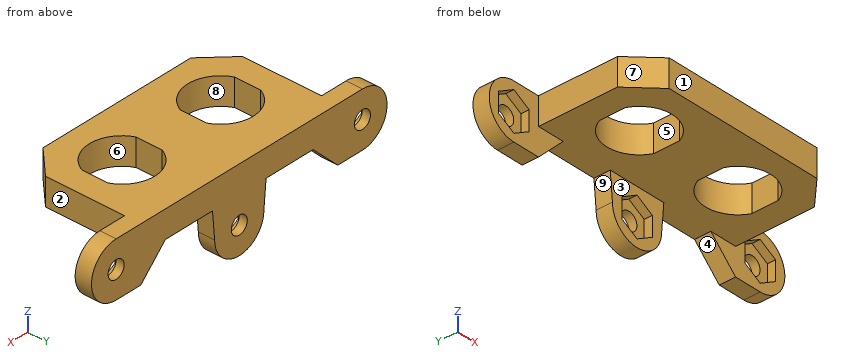
from build123d import *
from OCP.BRepFilletAPI import BRepFilletAPI_MakeChamfer

# Parameters (mm, degrees)
SKETCH1_R           = 1.625
BOSS_EXTRUDE1_DEPTH = 22.5
SKETCH5_W           = 15
SKETCH5_H           = 5
CUT_EXTRUDE1_DEPTH  = 41.388736054
CUT_EXTRUDE2_DEPTH  = 19.5
CUT_EXTRUDE3_DEPTH  = 39.810436741
CHAMFER1_SIZE       = 5
CHAMFER2_SIZE       = 0.437443318
CHAMFER2_SIZE_2     = 5
CHAMFER3_SIZE       = 5
CUT_EXTRUDE4_DEPTH  = 1.5


with BuildPart() as part:
    # Sketch1 → Boss-Extrude1 (new body)
    with BuildSketch(Plane(origin=(0, 0, 0), x_dir=(1, 0, 0), z_dir=(0, 1, 0))):
        with BuildLine():
            Line((-25, 10), (-5, 10))
            ThreePointArc((-5, 10), (0, 15), (5, 10))
            Line((5, 10), (25, 10))
            ThreePointArc((25, 10), (30, 5), (25, 0))
            Line((25, 0), (-25, 0))
            ThreePointArc((-25, 0), (-30, 5), (-25, 10))
        make_face()
        with Locations(Location((-25, 5, 0), (0, 0, 90))):
            Circle(SKETCH1_R, mode=Mode.SUBTRACT)
        with Locations(Location((25, 5, 0), (0, 0, 90))):
            Circle(SKETCH1_R, mode=Mode.SUBTRACT)
        with Locations(Location((0, 10, 0), (0, 0, 90))):
            Circle(SKETCH1_R, mode=Mode.SUBTRACT)
    extrude(amount=BOSS_EXTRUDE1_DEPTH)

    # Sketch5 → Cut-Extrude1 (cut, through all)
    with BuildSketch(Plane(origin=(0, 0, 0), x_dir=(1, 0, 0), z_dir=(0, 1, 0))):
        with Locations((-12.5, 7.5)):
            Rectangle(SKETCH5_W, SKETCH5_H)
        with Locations((12.5, 7.5)):
            Rectangle(SKETCH5_W, SKETCH5_H)
    extrude(amount=CUT_EXTRUDE1_DEPTH, mode=Mode.SUBTRACT)

    # Sketch6 → Cut-Extrude2 (cut)
    with BuildSketch(Plane.XZ):
        with BuildLine():
            Line((-25, 0), (-20, 0))
            Line((-20, 0), (-20, -10))
            Line((-20, -10), (-25, -10))
            ThreePointArc((-25, -10), (-30, -5), (-25, 0))
        make_face()
        with BuildLine():
            Line((20, 0), (20, -10))
            Line((20, -10), (25, -10))
            ThreePointArc((25, -10), (30, -5), (25, 0))
            Line((25, 0), (20, 0))
        make_face()
        with BuildLine():
            Line((-5, -5), (5, -5))
            Line((5, -5), (5, -10))
            ThreePointArc((5, -10), (0, -15), (-5, -10))
            Line((-5, -10), (-5, -5))
        make_face()
    extrude(amount=-CUT_EXTRUDE2_DEPTH, mode=Mode.SUBTRACT)

    # Sketch7 → Cut-Extrude3 (cut, through all)
    with BuildSketch(Plane(origin=(0, 0, -5), x_dir=(-1, 0, 0), z_dir=(0, 0, -1))):
        with BuildLine():
            Line((4.5, 12.397915762), (4.5, 7.602084238))
            ThreePointArc((4.5, 7.602084238), (10, 4), (15.5, 7.602084238))
            Line((15.5, 7.602084238), (15.5, 12.397915762))
            ThreePointArc((15.5, 12.397915762), (10, 16), (4.5, 12.397915762))
        make_face()
        with BuildLine():
            Line((-15.5, 12.397915762), (-15.5, 7.602084238))
            ThreePointArc((-15.5, 7.602084238), (-10, 4), (-4.5, 7.602084238))
            Line((-4.5, 7.602084238), (-4.5, 12.397915762))
            ThreePointArc((-4.5, 12.397915762), (-10, 16), (-15.5, 12.397915762))
        make_face()
    extrude(amount=-CUT_EXTRUDE3_DEPTH, mode=Mode.SUBTRACT)

    # Chamfer1
    chamfer1_edges = [part.edges().sort_by_distance(p)[0] for p in [
        (-20, 21, -5),
        (20, 21, -5),
    ]]
    chamfer(chamfer1_edges, length=CHAMFER1_SIZE - 0.0001)  # a hair under: the kernel refuses the full size

    # Chamfer2
    chamfer2_edges_1 = [part.edges().sort_by_distance(p)[0] for p in [
        (-5, 21, -5),
    ]]
    chamfer2_side_1 = [part.faces().sort_by_distance(p)[0] for p in [
        (-5.008748866, 21, -5),
    ]]
    chamfer2_edges_2 = [part.edges().sort_by_distance(p)[0] for p in [
        (5, 21, -5),
    ]]
    chamfer2_side_2 = [part.faces().sort_by_distance(p)[0] for p in [
        (5.008748866, 21, -5),
    ]]
    chamfer2 = BRepFilletAPI_MakeChamfer(part.part.solid().wrapped)
    for e in chamfer2_edges_1:
        chamfer2.Add(CHAMFER2_SIZE - 0.0001, CHAMFER2_SIZE_2 - 0.0001, e.wrapped, chamfer2_side_1[0].wrapped)
    for e in chamfer2_edges_2:
        chamfer2.Add(CHAMFER2_SIZE - 0.0001, CHAMFER2_SIZE_2 - 0.0001, e.wrapped, chamfer2_side_2[0].wrapped)
    add(Compound.cast(chamfer2.Shape()), mode=Mode.REPLACE)  # a hair under: the kernel refuses the full size

    # Chamfer3
    chamfer3_edges = [part.edges().sort_by_distance(p)[0] for p in [
        (-20, 0, -2.5),
        (20, 0, -2.5),
    ]]
    chamfer(chamfer3_edges, length=CHAMFER3_SIZE)

    # Sketch8 → Cut-Extrude4 (cut)
    with BuildSketch(Plane.XZ.offset(-19.5)):
        Polygon((25, -8.579571669), (28.1, -6.789785834), (28.1, -3.210214166), (25, -1.420428331), (21.9, -3.210214166), (21.9, -6.789785834), align=None)
        Polygon((0, -13.579571669), (3.1, -11.789785834), (3.1, -8.210214166), (0, -6.420428331), (-3.1, -8.210214166), (-3.1, -11.789785834), align=None)
        Polygon((-25, -8.579571669), (-21.9, -6.789785834), (-21.9, -3.210214166), (-25, -1.420428331), (-28.1, -3.210214166), (-28.1, -6.789785834), align=None)
    extrude(amount=-CUT_EXTRUDE4_DEPTH, mode=Mode.SUBTRACT)


solid = part.part
Design review of the part built by this model. Coordinates are the model's own, in mm. Face numbers are marked on the shaded views. A direction names the side the tool comes from. Round coordinates to 2 decimals unless told otherwise and drop trailing zeros. Order: outer loops, then holes, each group sorted by start corner. A loop starts at its lowest first (then second) coordinate and runs counter-clockwise, first axis right, second up.
1) Draft analysis for pull direction Y (two halves, no side actions). For the marked faces 6, 7, 8 and 9, state which applies: released by +Y, released by -Y, zero draft, split by the parting line, or undercut.
The answers:
face 6: undercut
face 7: released by -Y
face 8: undercut
face 9: zero draft
2) Clearance check with flat-ended pins moving along their axes: pin 1 Ø8 at (x, z) = (0.5, -7.5) entering from -Y; pin 2 Ø3 at (x, z) = (-22, -6) entering from -Y; pin 3 Ø6 at (x, y) = (21, 16) entering from -Z; pin 4 Ø2.5 at (y, z) = (10.5, -3.5) entering from -X. State where each tip first meets the part, or that it passes through.
The answers:
pin 1: stops at y = 0
pin 2: stops at y = 19.5
pin 3: stops at z = -5
pin 4: stops at x = -20
3) For L1, parallel to Z at x = 25, y = 21.85 (3 decimals); L2, parallel to X at y = 14, z = -2.75; L3, parallel to X at y = 14.25, z = -0.5, list the stretches that pass through material, from the lowest coordinate up.
The answers:
L1: z = -10 to -6.625, -3.375 to 0
L2: x = -20 to -14.47, -5.53 to 5.53, 14.47 to 20
L3: x = -20 to -14.24, -5.76 to 5.76, 14.24 to 20
4) Consider section C-C (x = -17.5). State the section outline as (y, z) points, plus the area to 4 significant figures.
The answers:
outline: (2.5, -5) - (19.5, -5) - (19.5, -7.5) - (22.5, -7.5) - (22.5, 0) - (2.5, 0) - close
area: 107.5 mm2
5) Consider section B-B (z = -12.5). State the section outline as (x, y) points.
The answers:
outline: (-4.33, 19.5) - (-1.87, 19.5) - (-1.87, 21) - (1.87, 21) - (1.87, 19.5) - (4.33, 19.5) - (4.33, 22.5) - (-4.33, 22.5) - close
6) Consider section A-A (x = 13.5). State the section outline as (y, z) points.
The answers:
outline: (0, -5) - (5.13, -5) - (5.13, 0) - (0, 0) - close; (14.87, -5) - (22.5, -5) - (22.5, 0) - (14.87, 0) - close
7) Machinability: for the marked faces 1, 2, 3, 4 and 5, which of the approach directions +Z, -Z, +X, -X, +Y, -Y give a long, thin tool a straight path to every point of the face, cutting with its end or side? Answer none if there is none.
The answers:
face 1: +Z, -Z, +X, -X, -Y
face 2: +Z, -Z, +X, -Y
face 3: -Z, +X, -X, -Y
face 4: -Z, +Y, -Y
face 5: +Z, -Z
